Read the model definition and answer for the solid it produces. Units are mm, in the model's axes. Face numbers are marked on the shaded views. A direction names the side the tool comes from. Give positions to 0.01 mm unless a question says otherwise; leave off trailing zeros. Order: outer loops, then holes, each group sorted by start corner. A loop starts at its lowest first (then second) coordinate and runs counter-clockwise, first axis right, second up. Notation, with made-up numbers: (38.5, -29) - (70.5, -29) arc R29 ccw to (70.5, 6) - close; hole circle Ø6 at (46.5, 67). An arc over 180 degrees is marked (long way). Write item = value, one per line.
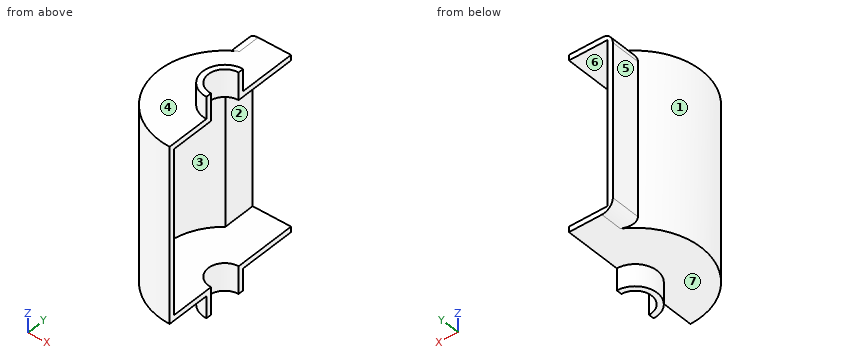
```python
from build123d import *

# Parameters (mm, degrees)
DODANIE_WYCI_GNI_CIE1_DEPTH       = 25
DODANIE_WYCI_GNI_CIE2_DEPTH       = 5
WYCI_GNI_CIE_CIENKA_START         = -150
WYCI_GNI_CIE_CIENKA_CIANKA2_DEPTH = 150
ZAOKR_GLENIE1_R                   = 10


with BuildPart() as part:
    # Szkic1 → Dodanie-wyci_gni_cie1 (new body)
    with BuildSketch(Plane.XY):
        with BuildLine():
            Line((0, 20), (0, 15))
            ThreePointArc((0, 15), (-15, 0), (0, -15))
            Line((0, -15), (0, -20))
            ThreePointArc((0, -20), (-20, 0), (0, 20))
        make_face()
    extrude(amount=DODANIE_WYCI_GNI_CIE1_DEPTH)

    # Szkic2 → Dodanie-wyci_gni_cie2 (add)
    with BuildSketch(Plane.XY):
        with BuildLine():
            Line((0, -20), (0, -60))
            ThreePointArc((0, -60), (-56.050341538, -21.409325386), (-40, 44.72135955))
            Line((-40, 44.72135955), (-40, 72))
            Line((-40, 72), (0, 72))
            Line((0, 72), (0, 20))
            ThreePointArc((0, 20), (-20, 0), (0, -20))
        make_face()
    extrude(amount=DODANIE_WYCI_GNI_CIE2_DEPTH)


with BuildPart() as body_2:
    # Lustro1: mirrored copy
    add(part.part.mirror(Plane.XY.offset(-75)))


with BuildPart() as part_1:
    add(part.part)

    add(body_2.part)  # Wyci_gni_cie-cienka _cianka2 merges body 2
    # Szkic3 → Wyci_gni_cie-cienka _cianka2 (add)
    with BuildSketch(Plane.XY.offset(WYCI_GNI_CIE_CIENKA_START)):
        with BuildLine():
            Line((-40, 72), (-40, 44.72135955))
            ThreePointArc((-40, 44.72135955), (-56.050341538, -21.409325386), (0, -60))
            Line((0, -60), (0, -55))
            ThreePointArc((0, -55), (-51.76124215, -18.594994247), (-35, 42.426406871))
            Line((-35, 42.426406871), (-35, 72))
            Line((-35, 72), (-40, 72))
        make_face()
    extrude(amount=WYCI_GNI_CIE_CIENKA_CIANKA2_DEPTH)

    # Zaokr_glenie1
    zaokr_glenie1_edges = [part_1.edges().sort_by_distance(p)[0] for p in [
        (-40, 58.360679775, 5),
        (-40, 58.360679775, -155),
    ]]
    fillet(zaokr_glenie1_edges, radius=ZAOKR_GLENIE1_R)


solid = part_1.part
```
1. Section B-B (z = -116) is taken. Determine the outline of the cut face in (x, y), and give its area (3 significant figures).
Recorded:
outline = (-40, 44.72) arc R60 ccw to (0, -60) - (0, -55) arc R55 cw to (-35, 42.43) - (-35, 72) - (-40, 72) - close
area = 841 mm^2
2. Section A-A (x = -51) is taken. Determine the outline of the cut face in (y, z).
Recorded:
outline = (-31.61, -155) - (31.61, -155) - (31.61, 5) - (-31.61, 5) - close; hole (-20.59, -150) - (20.59, -150) - (20.59, 0) - (-20.59, 0) - close
3. Section C-C (y = 0) is taken. Determine the outline of the cut face in (x, z).
Recorded:
outline = (-60, -155) - (-20, -155) - (-20, -175) - (-15, -175) - (-15, -150) - (-55, -150) - (-55, 0) - (-15, 0) - (-15, 25) - (-20, 25) - (-20, 5) - (-60, 5) - close
4. Straight lines are drawn through the part: L1, parallel to Z at x = -36.5, y = -9.5; L2, parallel to Z at x = -40, y = -38; L3, parallel to X at y = 49, z = -76.5. For each, find the intervals that lie inside material, in ascending order. Write a range as [from, to].
Recorded:
L1 = [-155, -150], [0, 5]
L2 = [-155, 5]
L3 = [-40, -35]
5. Flat-ended cylindrical pins translate along their axes: pin 1 (3 mm diameter, centred on x = -11, z = -97, fed in from +Y); pin 2 (8 mm diameter, centred on y = 56, z = -68, fed in from -X); pin 3 (6 mm diameter, centred on x = -51.5, z = -36.5, fed in from +Y). Find the tip coordinate at first contact, or state that the pin passes through.
Recorded:
pin_1 = -53.56
pin_2 = -40
pin_3 = 35.32
6. Section D-D (x = -38) is taken. Determine the outline of the cut face in (y, z).
Recorded:
outline = (-46.43, -155) - (46.43, -155) - (46.43, -151) - (72, -151) - (72, 1) - (46.43, 1) - (46.43, 5) - (-46.43, 5) - close; hole (-39.76, -150) - (39.76, -150) - (39.76, 0) - (-39.76, 0) - close
7. For the marked faces 4, 5, 6 and 7, determine the directions among +Z, -Z, +X, -X, +Y, -Y from which every point of the face is accessible in a straight line to the end or side of a thin tool.
Recorded:
face_4 = +Z, -X
face_5 = +Z, -Z, -X, +Y
face_6 = +X
face_7 = -Z, -X
8. Determine the mould class of the marked faces 1, 2 and 3 for opening direction Y: +Y half, -Y half, draft (parallel to the pull), parting line (faces both ways), or undercut.
Recorded:
face_1 = parting line
face_2 = draft
face_3 = undercut
